Here's how the part is built. I have some questions about the finished solid (model axes, mm). A direction names the side the tool comes from. Round coordinates to 2 decimals unless told otherwise and drop trailing zeros. Write each loop counter-clockwise with the first axis right and the second up, starting at its lowest first coordinate (ties: lowest second). Pieces come first, ordered by that corner, then holes. Notation, with made-up numbers: (16, 86.5) - (51, 86.5) arc R18 cw to (51, 94.5) - close; hole circle Ø2 at (44, 87). An arc over 180 degrees is marked (long way). Use one line per item in the form item = value. Start each with the question number.
1. Will these pins go through, and if not, where does the flat tip stop? pin 1 (3 mm diameter, centred on x = -319.8, y = -170.25, fed in from +Z); pin 2 (7.5 mm diameter, centred on x = -318.5, y = -156, fed in from +Z); pin 3 (10 mm diameter, centred on x = -67, y = -73.5, fed in from +Z); pin 4 (1.5 mm diameter, centred on x = -167, z = 501.5, fed in from -Y).
2. We'd pull the mould along X, two halves only. Please class faces 3 (the flat face through (-0.25, -197, 599)), 4 (the flat face through (-197, 0, 345)), 5 (the flat face through (0, -203, 345)): +X half, -X half, draft (parallel to the pull), parting line (faces both ways), or undercut.
3. If I drill on line 1 along X through (y, z) = (-366.5, 548); line 2 along X through (y, z) = (-170.25, 281.5); line 3 along Z through (x, y) = (-69, -58), over which ranges is the centre line in solid material (lowest first)?
4. I want a section at C-C, the plane y = -91. List the corners of the cut face in (x, z) for me.
5. I want a section at A-A, the plane x = -166. List the corners of the cut face in (y, z) for me.
6. I want a section at B-B, the plane y = -320. List the corners of the cut face in (x, z) for me.
7. Which directions (+Z, -Z, +X, -X, +Y, -Y) give clear straight access to the entire face, cutting with the end or side of a thin tool? Please do faces 1 (the flat face through (-203, -197, 0)), 2 (the flat face through (-399.75, -203, 599)).
```python
from build123d import *

# Parameters (mm, degrees)
F0_W     = 400
F0_H     = 500
F1_DEPTH = 400
F3_DEPTH = 200
F4_W     = 309.5
F4_H     = 200
F5_DEPTH = 1
F6_DEPTH = 5
F8_R     = 3.5
F9_DEPTH = 9
F11_D    = 5
F13_D    = 5


with BuildPart() as f1:
    # F0 (on Front) → F1 (new body)
    with BuildSketch(Plane.XZ):
        with Locations((-200, 250)):
            Rectangle(F0_W, F0_H)
    extrude(amount=F1_DEPTH)

    # F2 (on face) → F3 (join)
    with BuildSketch(Plane.XY.offset(500)):
        Polygon((-399.75, 0), (-400, 0), (-400, -0.25), (-400, -400), (-399.75, -400), (-399.75, -0.25), (-0.25, -0.25), (-0.25, -400), (0, -400), (0, -0.25), (0, 0), (-0.25, 0), align=None)
    extrude(amount=F3_DEPTH)

    # F4 (on face) → F5 (join)
    with BuildSketch(Plane.XY.offset(500)):
        with Locations((-200, -175.25)):
            Rectangle(F4_W, F4_H)
    extrude(amount=F5_DEPTH)

    # F4 (on face) → F6 (join)
    with BuildSketch(Plane.XY.offset(500)):
        with Locations((-200, -175.25)):
            Rectangle(F4_W, F4_H)
    extrude(amount=F6_DEPTH)

    # F8 (on face) → F9 (join)
    with BuildSketch(Plane.XY.offset(505)):
        with Locations((-319.801312, -155.25)):
            Circle(F8_R)
        with Locations((-319.801312, -170.25)):
            Circle(F8_R)
    extrude(amount=F9_DEPTH)

    # F11 (through all)
    with Locations(Plane.XY.offset(514)):
        with Locations((-319.801312, -155.25)):
            Hole(F11_D / 2)

    # F13 (through all)
    with Locations(Plane.XY.offset(514)):
        with Locations((-319.801312, -170.25)):
            Hole(F13_D / 2)


solid = f1.part
```
Model answer:
q1.pin_1 = through
q1.pin_2 = 514
q1.pin_3 = 505
q1.pin_4 = -275.25
q2.face_3 = undercut
q2.face_4 = draft
q2.face_5 = +X half
q3.line_1 = -400 to -399.75, -0.25 to 0
q3.line_2 = -400 to -322.3, -317.3 to 0
q3.line_3 = 0 to 500
q4.outline = (-400, 0) - (0, 0) - (0, 700) - (-0.25, 700) - (-0.25, 500) - (-45.25, 500) - (-45.25, 505) - (-354.75, 505) - (-354.75, 500) - (-399.75, 500) - (-399.75, 700) - (-400, 700) - close
q5.outline = (-400, 0) - (0, 0) - (0, 700) - (-0.25, 700) - (-0.25, 500) - (-75.25, 500) - (-75.25, 505) - (-275.25, 505) - (-275.25, 500) - (-400, 500) - close
q6.outline = (-400, 0) - (0, 0) - (0, 700) - (-0.25, 700) - (-0.25, 500) - (-399.75, 500) - (-399.75, 700) - (-400, 700) - close
q7.face_1 = -Z, +X, -X, +Y, -Y
q7.face_2 = +Z, -Y
